Can you work these out from the drawing? Everything is in mm from the part's minimum corner. Round coordinates to 2 decimals unless told otherwise and drop trailing zeros. Write each loop counter-clockwise with the first axis right and the second up, starting at its lowest first coordinate (ties: lowest second). Pieces come first, ordered by that corner, then holes. Notation, with made-up numbers: M -8.5,0 L 32.5,0 A19 cw 32.5,23 Z; hole C 14.25,42 d4. An arc over 180 degrees is marked long. Use one line per item in the form item = value. Start each with the question number.
Q1. I want a section at B-B on z = 1.8. List the corners of the cut face in (x, y) for me, and give its area (3 significant figures).
Q2. I'm going to push flat-ended pins straight in: pin 1 Ø6 at (x, y) = (12, 71) entering from -Z; pin 2 Ø4.5 at (x, y) = (5, 85) entering from -Z. Where does each tip first touch, or does it pass through?
Q3. I want a section at C-C on y = 85. List the corners of the cut face in (x, z) for me, and give its area (3 significant figures).
Q4. I want a section at D-D on x = 4.5. List the corners of the cut face in (y, z) for me, and give its area (3 significant figures).
Q5. I want a section at A-A on x = 23.24. List the corners of the cut face in (y, z) for me.
Q6. I need wall thicknesses on line 1 along X through (y, z) = (85, 0.8); line 2 along Y through (x, z) = (5, 1.45); line 3 along Y through (x, z) = (3.75, 2.25). Which ranges of each line are inside material? Lowest first, please. Write a range as from..to.
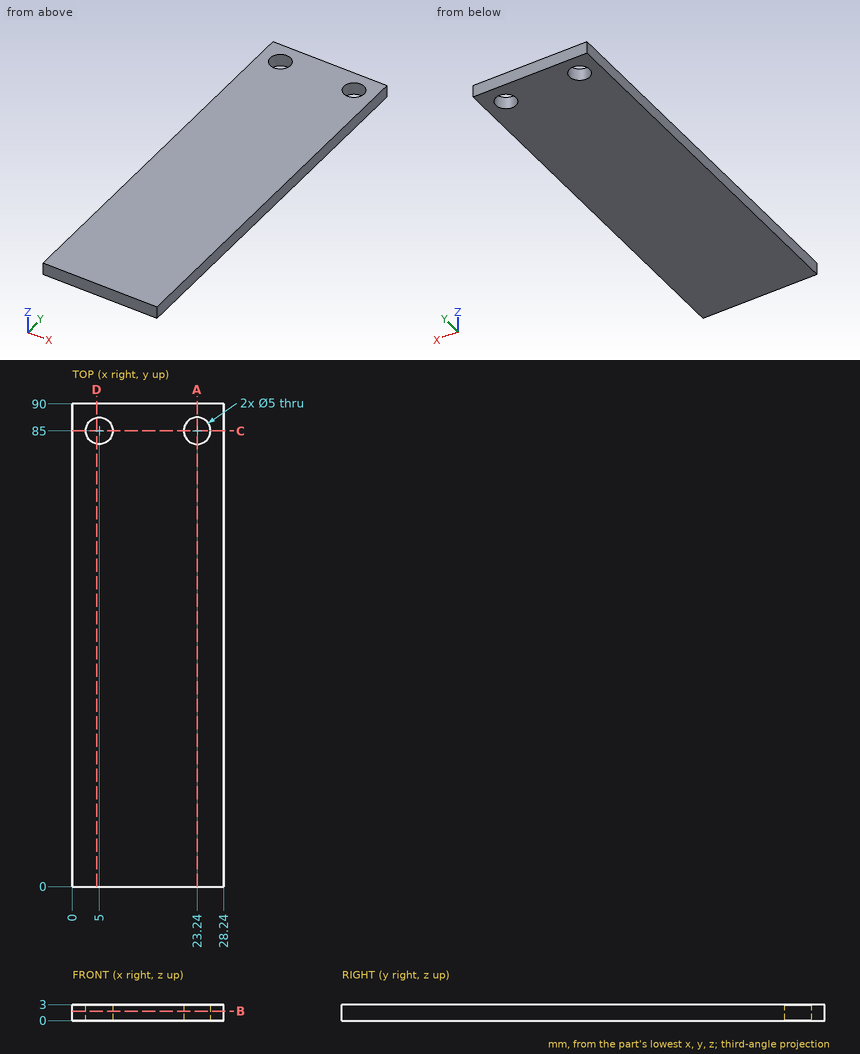
Reported:
q1.outline = M 0,0 L 28.24,0 L 28.24,90 L 0,90 Z; hole C 5,85 d5; hole C 23.24,85 d5
q1.area = 2,500 mm^2
q2.pin_1 = 0
q2.pin_2 = through
q3.outline = M 0,0 L 2.5,0 L 2.5,3 L 0,3 Z; M 7.5,0 L 20.74,0 L 20.74,3 L 7.5,3 Z; M 25.74,0 L 28.24,0 L 28.24,3 L 25.74,3 Z
q3.area = 54.7 mm^2
q4.outline = M 0,0 L 82.55,0 L 82.55,3 L 0,3 Z; M 87.45,0 L 90,0 L 90,3 L 87.45,3 Z
q4.area = 255 mm^2
q5.outline = M 0,0 L 82.5,0 L 82.5,3 L 0,3 Z; M 87.5,0 L 90,0 L 90,3 L 87.5,3 Z
q6.line_1 = 0..2.5, 7.5..20.74, 25.74..28.24
q6.line_2 = 0..82.5, 87.5..90
q6.line_3 = 0..82.83, 87.17..90
